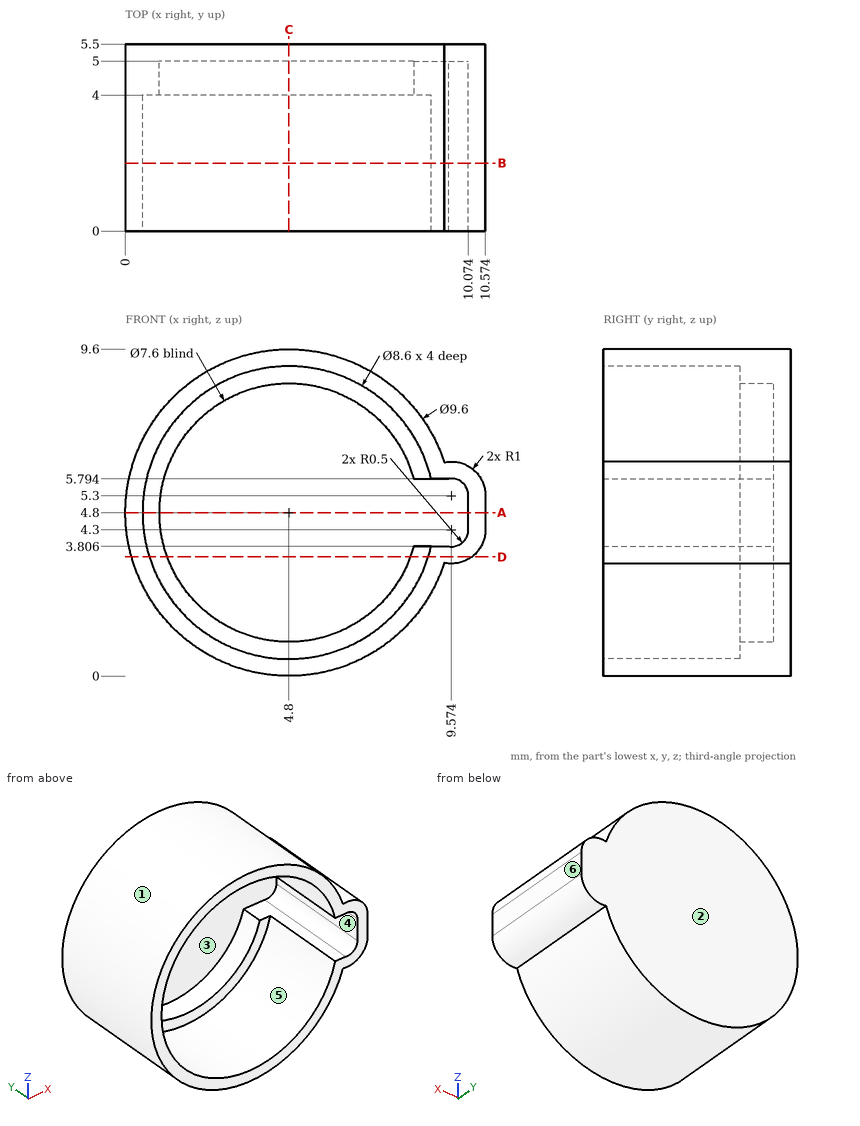
Check sheet for the drawn part. Datum: minimum x, y, z corner. Units: mm. A direction names the side the tool comes from. Give positions to 0.01 mm unless a question says otherwise; leave off trailing zeros. Write each loop counter-clockwise with the first axis right and the second up, starting at its lowest first coordinate (ties: lowest second). Pieces come first, ordered by that corner, then holes.
(1) Mould release check, pull along X, two halves, no side actions. Record for the marked faces 1, 2, 3 and 4: +X half, -X half, draft (parallel to the pull), parting line (faces both ways), or undercut.
(2) Cross-section at C-C (x = 4.8). Enter the section's corners in (y, z), plus the area to 3 significant figures.
(3) Cross-section at B-B (y = 2). Enter the section's corners in (x, z), plus the area to 3 significant figures.
(4) Gauge pin test, flat ends, axial feed: pin 1 (1.5 mm diameter, centred on y = 2, z = 8.5, fed in from +X); pin 2 (0.8 mm diameter, centred on x = 9, y = 2.5, fed in from +Z); pin 3 (3 mm diameter, centred on x = 9.5, y = 1.5, fed in from +Z). Record the tip position at first contact, or that the pin passes through.
(5) Cross-section at D-D (z = 3.5). Enter the section's corners in (x, y), plus the area to 3 significant figures.
(6) Access from +Z, -Z, +X, -X, +Y, -Y to the whole of each face (thin tool, end or side, straight path). Record for the marked faces 5 and 6.
(7) Material ranges on line 1 (Z direction, x = 4.8, y = 4.75); line 2 (X direction, y = 4.8, z = 4.8); line 3 (Z direction, x = 4.8, y = 1.7), recorded low to high.
(8) Cross-section at A-A (z = 4.8). Enter the section's corners in (x, y), plus the area to 3 significant figures.
Worked out:
1. face 1: parting line
1. face 2: draft
1. face 3: undercut
1. face 4: undercut
2. outline: (0, 0) - (5.5, 0) - (5.5, 9.6) - (0, 9.6) - (0, 9.1) - (4, 9.1) - (4, 8.6) - (5, 8.6) - (5, 1) - (4, 1) - (4, 0.5) - (0, 0.5) - close
2. area: 10.8 mm2
3. outline: (9.37, 3.32) arc R1 ccw to (10.57, 4.3) - (10.57, 5.3) arc R1 ccw to (9.37, 6.28) arc R4.8 ccw (long way) to start; hole (8.98, 3.81) - (9.5, 3.81) arc R0.5 ccw to (10.07, 4.3) - (10.07, 5.3) arc R0.5 ccw to (9.5, 5.79) - (8.98, 5.79) arc R4.3 ccw (long way) to start
3. area: 15.1 mm2
4. pin 1: stops at x = 8.59
4. pin 2: stops at z = 7.73
4. pin 3: stops at z = 8.38
5. outline: (0.18, 0) - (0.7, 0) - (0.7, 4) - (1.23, 4) - (1.23, 5) - (8.37, 5) - (8.37, 4) - (8.9, 4) - (8.9, 0) - (10.17, 0) - (10.17, 5.5) - (0.18, 5.5) - close
5. area: 15.0 mm2
6. face 5: -Y
6. face 6: +Z, -Z, +X, +Y, -Y
7. line 1: z = 0 to 1, 8.6 to 9.6
7. line 2: x = 0 to 1, 10.07 to 10.57
7. line 3: z = 0 to 0.5, 9.1 to 9.6
8. outline: (0, 0) - (0.5, 0) - (0.5, 4) - (1, 4) - (1, 5) - (10.07, 5) - (10.07, 0) - (10.57, 0) - (10.57, 5.5) - (0, 5.5) - close
8. area: 10.8 mm2
